from build123d import *

# Parameters (mm, degrees)
F0_W     = 20
F0_H     = 50
F0_H_2   = 2
F1_DEPTH = 8
F3_DEPTH = 50
F4_DEPTH = 25.4
F5_T     = -2
F6_W     = 2
F6_H     = 4
F6_H_2   = 2
F6_W_2   = 20
F6_W_3   = 43.6544959545
F7_DEPTH = 8


with BuildPart() as f1:
    # F0 (on Front) → F1 (new body)
    with BuildSketch(Plane.XZ):
        Polygon((12, 27), (-12, 27), (-12, -27), (-10, -27), (-10, -25), (-10, 25), (10, 25), (10, -25), (10, -27), (12, -27), align=None)
        Rectangle(F0_W, F0_H)
        with Locations((0, -26)):
            Rectangle(F0_W, F0_H_2)
    extrude(amount=F1_DEPTH)

    # F2 (on Right) → F3 (cut)
    with BuildSketch(Plane.YZ):
        Polygon((-6.5, 23.2472232503), (-1.5, 26.1339745962), (0, 27), (-8, 27), (-8, 22.3811978465), align=None)
    extrude(amount=-F3_DEPTH, mode=Mode.SUBTRACT)

    # F2 (on Right) → F4 (cut)
    with BuildSketch(Plane.YZ):
        Polygon((-6.5, 23.2472232503), (-1.5, 26.1339745962), (0, 27), (-8, 27), (-8, 22.3811978465), align=None)
    extrude(amount=F4_DEPTH, mode=Mode.SUBTRACT)

    # F5
    f5_openings = [f1.faces().sort_by_distance(p)[0] for p in [
        (0, 0, 0),
        (0, -4, -27),
    ]]
    offset(amount=F5_T, openings=f5_openings)

    # F6 (on face) → F7 (join)
    with BuildSketch(Plane(origin=(0, 0, 0), x_dir=(-1, 0, 0), z_dir=(0, 1, 0))):
        with Locations((11, -29)):
            Rectangle(F6_W, F6_H)
        with Locations((11, -32)):
            Rectangle(F6_W, F6_H_2)
        Polygon((10, -31), (10, -27), (-10, -27), (-10, -29), (-53.6544959545, -29), (-53.6544959545, -31), (-10, -31), align=None)
        with Locations((0, -32)):
            Rectangle(F6_W_2, F6_H_2)
        Polygon((-10, -29), (-10, -27), (-12, -27), (-53.6544959545, -27), (-53.6544959545, -29), align=None)
        with Locations((-31.8272479773, -32)):
            Rectangle(F6_W_3, F6_H_2)
        with Locations((-54.6544959545, -32)):
            Rectangle(F6_W, F6_H_2)
        with Locations((-54.6544959545, -30)):
            Rectangle(F6_W, F6_H_2)
        with Locations((-54.6544959545, -28)):
            Rectangle(F6_W, F6_H_2)
    extrude(amount=-F7_DEPTH)


solid = f1.part
For this review, take the finished solid that the model builds, in its own axes (mm). A direction names the side the tool comes from. Round coordinates to 2 decimals unless told otherwise and drop trailing zeros. Order: outer loops, then holes, each group sorted by start corner. A loop starts at its lowest first (then second) coordinate and runs counter-clockwise, first axis right, second up. Notation, with made-up numbers: M 13.25,87 L 42.25,87 A19 ccw 42.25,118 Z; hole C 0,5.25 d1. An arc over 180 degrees is marked long. Use a Markdown table: item, result. Add a question column.
Item 1: Add section A-A, the plane y = -4. Give the boundary of the cut face in (x, z).
Item 2: Tool access review of faces 1 (the flat face through (12, -4, 0)), 2 (the flat face through (0, -3, -27)), 3 (the flat face through (-12, -4, -3)): name each direction out of +Z, -Z, +X, -X, +Y, -Y from which nothing blocks a thin tool from reaching the whole face with its end or side.
Item 3: Add section B-B, the plane z = -2. Give the boundary of the cut face in (x, y).
Item 4: Mouldability with a two-part tool opening along Z and no side actions: class faces 4 (the flat face through (55.654, -4, -30)), 5 (the flat face through (0, -6, -3)), 6 (the flat face through (22, -4, -33)) as released by +Z, released by -Z, zero draft, split by the parting line, or undercut.
Item 5: Insertion check: pin 1 (12 mm diameter, centred on x = 20.5, z = 9.5, fed in from +Y); pin 2 (4 mm diameter, centred on x = -1, z = -19, fed in from +Y); pin 3 (4 mm diameter, centred on x = 35.5, y = -4.5, fed in from +Z); pin 4 (3 mm diameter, centred on x = 4, y = -3, fed in from +Z). Each pin has a flat end and moves straight along its axis. Give the tip position at first contact, or say it passes through.
Item 6: Add section C-C, the plane x = -4.5. Give the boundary of the cut face in (y, z).
Item 7: Add section D-D, the plane x = 45. Give the boundary of the cut face in (y, z).
Item 8: To check wall thickness, follow line 1 along X through (y, z) = (-1, -19.5); line 2 along Z through (x, y) = (20, -7.25); line 3 along X through (y, z) = (-6.75, 19). State the ranges of each line that lie inside material, in increasing order.
Geometry results:
| question | item | result |
|---|---|---|
| 1 | outline | M -12,-33 L 55.65,-33 L 55.65,-27 L 12,-27 L 12,24.69 L -12,24.69 Z; hole M -10,-27 L 10,-27 L 10,22.38 L -10,22.38 Z |
| 2 | face 1 | +Z, +X, +Y, -Y |
| 2 | face 2 | +Y |
| 2 | face 3 | +Z, -Z, -X, +Y, -Y |
| 3 | outline | M -12,-8 L 12,-8 L 12,0 L 10,0 L 10,-6 L -10,-6 L -10,0 L -12,0 Z |
| 4 | face 4 | zero draft |
| 4 | face 5 | undercut |
| 4 | face 6 | released by -Z |
| 5 | pin 1 | passes through |
| 5 | pin 2 | stops at y = -6 |
| 5 | pin 3 | stops at z = -27 |
| 5 | pin 4 | stops at z = 26.13 |
| 6 | outline | M -8,-33 L 0,-33 L 0,-27 L -6,-27 L -6,21.23 L 0,24.69 L 0,27 L -8,22.38 Z |
| 7 | outline | M -8,-33 L 0,-33 L 0,-27 L -8,-27 Z |
| 8 | line 1 | x = -12 to -10, 10 to 12 |
| 8 | line 2 | z = -33 to -27 |
| 8 | line 3 | x = -12 to 12 |
